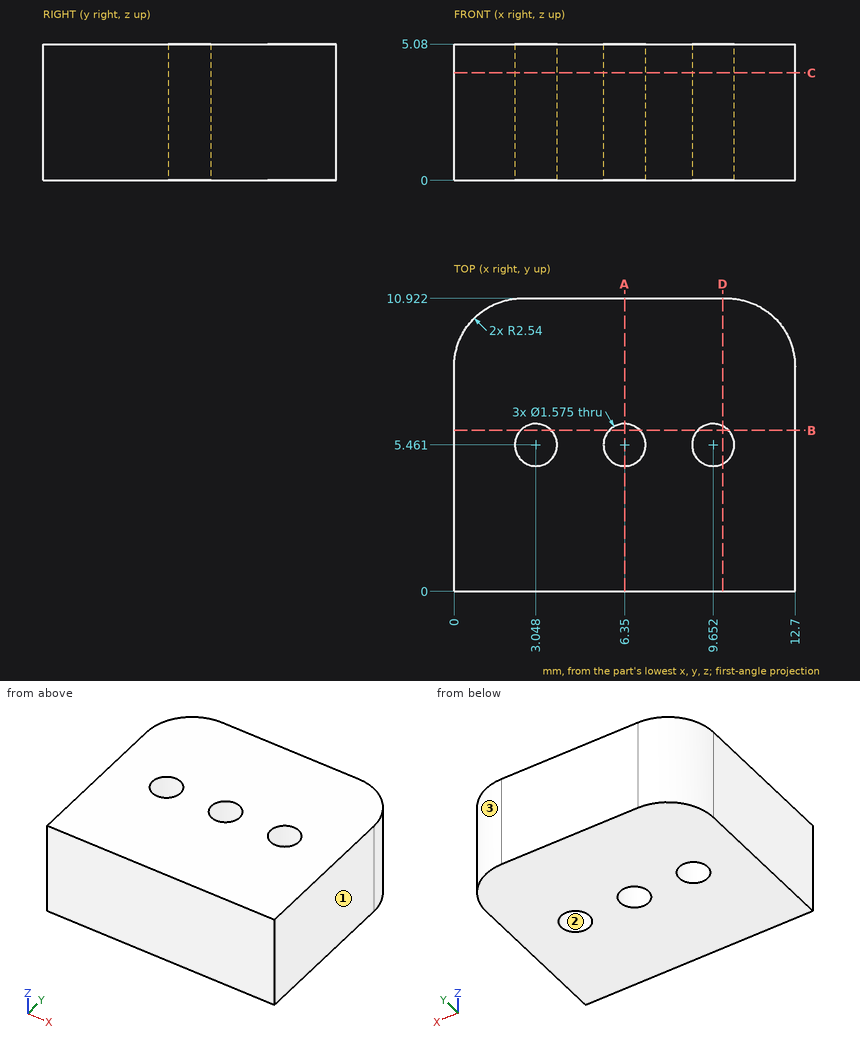
Here's the drawing with two shaded views (mm, measured from the low corner). I have some questions. Give positions to 0.01 mm unless a question says otherwise; leave off trailing zeros. Write each loop counter-clockwise with the first axis right and the second up, starting at its lowest first coordinate (ties: lowest second). Pieces come first, ordered by that corner, then holes. Notation, with made-up numbers: (-33.75, 74.5) -> (20.25, 74.5) arc R12 ccw to (20.25, 93.5) -> close; hole circle Ø10 at (-40, 63). An arc over 180 degrees is marked (long way). Answer as a JSON object with one key per item and string values. Group by question number.
Item 1: Please list where these lines run through material, in increasing order: line 1 (X direction, y = 5, z = 4.8); line 2 (Y direction, x = 9.75, z = 4.7); line 3 (Y direction, x = 10, z = 3.75) (1 decimal). Write a range as [from, to].
Item 2: Suppose I cut it at D-D (x = 10). Please give me the cut outline in (y, z) (1 decimal).
Item 3: Suppose I cut it at B-B (y = 6). Please give me the cut outline in (x, z).
Item 4: I'm going to push a flat-ended pin straight in: P1, Ø1.4, axis at x = 9.652, y = 5.461, coming from the +Z side. Where does the tip first touch, or does it pass through?
Item 5: Suppose I cut it at C-C (z = 4). State how many separate pieces and enclosed holes the cut face has, plus the area to 3 significant figures.
Item 6: Suppose I cut it at A-A (x = 6.35). Please give me the cut outline in (y, z).
Item 7: We'd pull the mould along Y, two halves only. Please class the marked faces 1, 2 and 3: +Y half, -Y half, draft (parallel to the pull), parting line (faces both ways), or undercut.
Findings:
{
 "1": {"line 1": "x = [0, 2.41], [3.69, 5.71], [6.99, 9.01], [10.29, 12.7]", "line 2": "y = [0, 4.68], [6.24, 10.92]", "line 3": "y = [0, 4.8], [6.2, 10.9]"},
 "2": {"outline": "(0, 0) -> (4.8, 0) -> (4.8, 5.1) -> (0, 5.1) -> close; (6.2, 0) -> (10.9, 0) -> (10.9, 5.1) -> (6.2, 5.1) -> close"},
 "3": {"outline": "(0, 0) -> (2.47, 0) -> (2.47, 5.08) -> (0, 5.08) -> close; (3.62, 0) -> (5.78, 0) -> (5.78, 5.08) -> (3.62, 5.08) -> close; (6.92, 0) -> (9.08, 0) -> (9.08, 5.08) -> (6.92, 5.08) -> close; (10.23, 0) -> (12.7, 0) -> (12.7, 5.08) -> (10.23, 5.08) -> close"},
 "4": {"P1": "passes through"},
 "5": {"separate pieces": "1", "enclosed holes": "3", "area": "130 mm²"},
 "6": {"outline": "(0, 0) -> (4.67, 0) -> (4.67, 5.08) -> (0, 5.08) -> close; (6.25, 0) -> (10.92, 0) -> (10.92, 5.08) -> (6.25, 5.08) -> close"},
 "7": {"face 1": "draft", "face 2": "undercut", "face 3": "+Y half"}
}
